Geometry: final body of the model. Coordinates: model frame, mm. A direction names the side the tool comes from. Give positions to 0.01 mm unless a question says otherwise; leave off trailing zeros. One line per question, with ' | ' between items. Start each with the question number.
(1) Ray query, L1, parallel to Y at x = 0, z = 22.5 (3 decimals); L2, parallel to Y at x = 0, z = 10.5 (1 decimal); L3, parallel to X at y = -2.5, z = 23. Return the intervals inside material, ascending.
(2) First-contact query: pin 1 Ø8 at (x, z) = (5.5, 14.5) entering from +Y; pin 2 Ø4 at (y, z) = (-2.5, 7.5) entering from +X; pin 3 Ø5.5 at (y, z) = (0, 18.669) entering from -X. Flat tips, straight axial feed; report the tip coordinate or a pass-through.
(3) Set-up query: faces 5 (the face through (-0.719, 5.477, 5.447)), 6 (the face through (13.07, 0.24, 24.19)), 7 (the face through (18.669, -2, 16)), 8 (the face through (5.239, 1.248, 14.706)), 9 (the face through (-0.719, 5.477, 31.891)). Return all of +Z, -Z, +X, -X, +Y, -Y with unobstructed straight access to the full face (end or side cutting, diameter ignored); none if empty.
(4) Section B-B (y = 0). State how many separate pieces and enclosed holes the cut face has, then the cut area to 3 significant figures.
(5) Mould query, pull axis Z, two halves, no side actions, for faces 1 (the face through (2.4, -2.4, 37.338)), 2 (the face through (3.63, 2.75, 21.66)), 3 (the face through (2.4, -2.4, 0)), 4 (the face through (10.34, 0.14, 21.84)). Classes: +Z half, -Z half, draft (parallel to the pull), parting line (faces both ways), or undercut.
```python
from build123d import *

# Parameters (mm, degrees)
SKETCH1_R           = 5.5245
BOSS_EXTRUDE1_DEPTH = 11.049
SKETCH2_R           = 4.064
BOSS_EXTRUDE2_DEPTH = 5.08
SKETCH3_R           = 5.5245
SKETCH4_R           = 4.064
SKETCH5_R           = 4.064
BOSS_EXTRUDE3_DEPTH = 5.08
SKETCH6_R           = 5.5245
BOSS_EXTRUDE4_DEPTH = 11.049
SKETCH7_R           = 3.175
CUT_EXTRUDE1_DEPTH  = 16.891
SKETCH9_R           = 3.175
CUT_EXTRUDE2_DEPTH  = 49.403


with BuildPart() as part:
    # Sketch1 → Boss-Extrude1 (new body)
    with BuildSketch(Plane.XY):
        Circle(SKETCH1_R)
    boss_extrude1 = extrude(amount=BOSS_EXTRUDE1_DEPTH)



with BuildPart() as body_2:
    # Sketch2 → Boss-Extrude2 (new body)
    with BuildSketch(Plane.XY.offset(13.589)):
        Circle(SKETCH2_R)
    boss_extrude2 = extrude(amount=BOSS_EXTRUDE2_DEPTH)


with BuildPart() as part_1:
    add(part.part)

    add(body_2.part)  # Loft2 merges body 2
    # Sketch3 → Loft2 section 0
    with BuildSketch(Plane.XY.offset(11.049)):
        Circle(SKETCH3_R)
    # Sketch4 → Loft2 section 1
    with BuildSketch(Plane.XY.offset(13.589)):
        Circle(SKETCH4_R)
    loft2 = loft()

    # Mirror5: Boss-Extrude1, Boss-Extrude2, Loft2 across plane
    add(boss_extrude1.mirror(Plane.XY.offset(18.669)))
    add(boss_extrude2.mirror(Plane.XY.offset(18.669)))
    add(loft2.mirror(Plane.XY.offset(18.669)))

    # Sketch5 → Boss-Extrude3 (add)
    with BuildSketch(Plane(origin=(0, 0, 0), x_dir=(0, 0, -1), z_dir=(1, 0, 0))):
        with Locations((-18.669, 0)):
            Circle(SKETCH5_R)
    extrude(amount=BOSS_EXTRUDE3_DEPTH)



with BuildPart() as body_2_2:
    # Sketch6 → Boss-Extrude4 (new body)
    with BuildSketch(Plane(origin=(7.62, 0, 0), x_dir=(0, 0, -1), z_dir=(1, 0, 0))):
        with Locations((-18.669, 0)):
            Circle(SKETCH6_R)
    extrude(amount=BOSS_EXTRUDE4_DEPTH)


with BuildPart() as part_2:
    add(part_1.part)

    add(body_2_2.part)  # loft3 joins it to this body
    # loft up to a face of the part (loft3)
    loft([Face(Wire([part_2.edges().sort_by_distance((5.08, 2.962528502, 21.450999438))[0]])), Face(Wire([part_2.edges().sort_by_distance((7.62, -4.027187182, 22.450780487))[0]]))])

    # Sketch7 → Cut-Extrude1 (cut)
    with BuildSketch(Plane(origin=(18.669, 0, 0), x_dir=(0, 0, -1), z_dir=(1, 0, 0))):
        with Locations((-18.669, 0)):
            Circle(SKETCH7_R)
    extrude(amount=-CUT_EXTRUDE1_DEPTH, mode=Mode.SUBTRACT)

    # Sketch9 → Cut-Extrude2 (cut)
    with BuildSketch(Plane(origin=(0, 0, 0), x_dir=(-1, 0, 0), z_dir=(0, 0, -1))):
        Circle(SKETCH9_R)
    extrude(amount=-CUT_EXTRUDE2_DEPTH, mode=Mode.SUBTRACT)


solid = part_2.part
```
Response:
1) L1: y = -4.064 to -3.175, 3.175 to 4.064 | L2: y = -5.5 to -3.2, 3.2 to 5.5 | L3: x = -3.2 to -1.96, 1.96 to 3.2, 6.71 to 18.67
2) pin 1: stops at y = 5.47 | pin 2: stops at x = 5.5 | pin 3: stops at x = -4.06
3) face 5: -Z | face 6: +X | face 7: +Z, -Z, +X, +Y, -Y | face 8: none | face 9: +Z
4) separate pieces: 3 | enclosed holes: 0 | area: 195 mm^2
5) face 1: +Z half | face 2: undercut | face 3: -Z half | face 4: undercut
